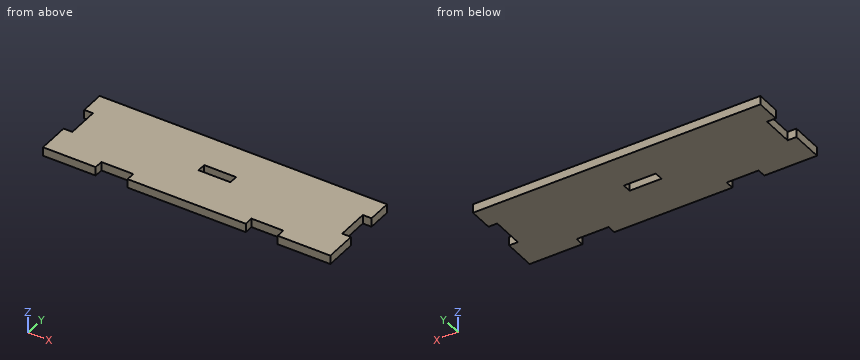
from build123d import *

# Parameters (mm, degrees)
BOSS_EXTRUDE1_DEPTH = 5.5
SKETCH3_W           = 20
SKETCH3_H           = 5.5
CUT_EXTRUDE2_DEPTH  = 5.5


with BuildPart() as part:
    # Sketch1 → Boss-Extrude1 (new body)
    with BuildSketch(Plane.XY):
        Polygon((0, 0), (33, 0), (33, 5.5), (53, 5.5), (53, 0), (127, 0), (127, 5.5), (147, 5.5), (147, 0), (180, 0), (180, 20), (174.5, 20), (174.5, 40), (180, 40), (180, 55), (0, 55), (0, 40), (5.5, 40), (5.5, 20), (0, 20), align=None)
    extrude(amount=BOSS_EXTRUDE1_DEPTH)

    # Sketch3 → Cut-Extrude2 (cut)
    with BuildSketch(Plane.XY.offset(5.5)):
        with Locations((90, 29.75)):
            Rectangle(SKETCH3_W, SKETCH3_H)
    extrude(amount=-CUT_EXTRUDE2_DEPTH, mode=Mode.SUBTRACT)


solid = part.part
The model under review builds one solid part; all positions refer to its coordinate system, in mm. Give positions to 0.01 mm unless a question says otherwise; leave off trailing zeros. Loops run counter-clockwise (first coordinate to the right, second up) from the corner with the lowest first, then second, coordinate; pieces in that order, holes last. Notation, with made-up numbers: (40, 21) -> (77, 21) arc R15 ccw to (77, 45) -> close; hole circle Ø10 at (68.5, 53). An arc over 180 degrees is marked (long way). Answer as a JSON object with one key per item and string values. Group by question number.
Q1. Wall thickness on line 1 along X through (y, z) = (4, 2.7); line 2 along Y through (x, z) = (92, 2.45); line 3 along X through (y, z) = (30, 1.35): over which ranges is each line inside the solid? List them lowest first.
Q2. Take a section at C-C (x = 138). Write out the cut boundary in (y, z).
Q3. Take a section at A-A (z = 4). Write out the cut boundary in (x, y), plus the area to 3 significant figures.
Q4. Insertion check: pin 1 (3 mm diameter, centred on x = 45, z = 3.5, fed in from -Y). The pin has a flat end and moves straight along its axis. Give the tip position at first contact, or say it passes through.
Q5. Take a section at B-B (y = 38). Write out the cut boundary in (x, z).
Answer below:
{
 "1": {"line 1": "x = 0 to 33, 53 to 127, 147 to 180", "line 2": "y = 0 to 27, 32.5 to 55", "line 3": "x = 5.5 to 80, 100 to 174.5"},
 "2": {"outline": "(5.5, 0) -> (55, 0) -> (55, 5.5) -> (5.5, 5.5) -> close"},
 "3": {"outline": "(0, 0) -> (33, 0) -> (33, 5.5) -> (53, 5.5) -> (53, 0) -> (127, 0) -> (127, 5.5) -> (147, 5.5) -> (147, 0) -> (180, 0) -> (180, 20) -> (174.5, 20) -> (174.5, 40) -> (180, 40) -> (180, 55) -> (0, 55) -> (0, 40) -> (5.5, 40) -> (5.5, 20) -> (0, 20) -> close; hole (80, 27) -> (100, 27) -> (100, 32.5) -> (80, 32.5) -> close", "area": "9,350 mm2"},
 "4": {"pin 1": "stops at y = 5.5"},
 "5": {"outline": "(5.5, 0) -> (174.5, 0) -> (174.5, 5.5) -> (5.5, 5.5) -> close"}
}
